Part model, mm, in its own coordinate system. Round coordinates to 2 decimals unless told otherwise and drop trailing zeros. Loops run counter-clockwise (first coordinate to the right, second up) from the corner with the lowest first, then second, coordinate; pieces in that order, holes last.
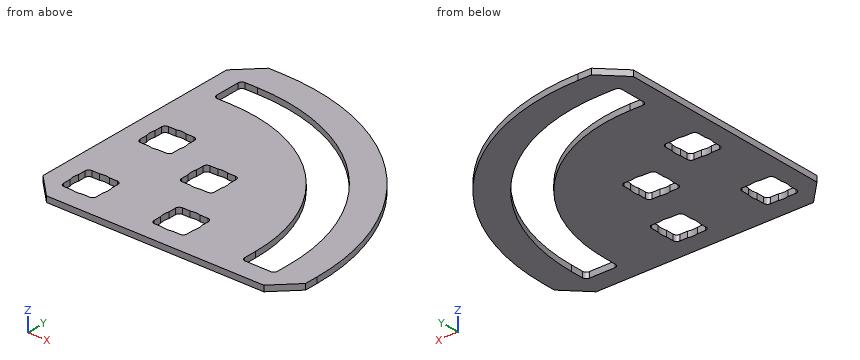
from build123d import *

# Parameters (mm, degrees)
BOSS_EXTRUDE1_DEPTH = 0.8128
SKETCH2_R           = 2.413
CUT_EXTRUDE1_DEPTH  = 2.54


with BuildPart() as part:
    # Sketch1 → Boss-Extrude1 (new body)
    with BuildSketch(Plane.XY.offset(0.8128)):
        with BuildLine():
            Line((-14.966560113, 23.146095061), (-14.966560113, -7.333904636))
            Line((-14.966560113, -7.333904636), (-11.791560113, -10.508904636))
            Line((-11.791560113, -10.508904636), (18.688439584, -10.508904636))
            Line((18.688439584, -10.508904636), (21.863439584, -7.333904636))
            Line((21.863439584, -7.333904636), (21.863439584, -5.428904939))
            ThreePointArc((21.863439584, -5.428904939), (12.564079886, 17.021735364), (-9.886560416, 26.321095061))
            Line((-9.886560416, 26.321095061), (-11.791560113, 26.321095061))
            Line((-11.791560113, 26.321095061), (-14.966560113, 23.146095061))
        make_face()
        with BuildLine():
            Line((17.316839733, -7.740304939), (13.710039804, -7.740304939))
            ThreePointArc((13.710039804, -7.740304939), (13.350829567, -7.591515187), (13.202039815, -7.23230495))
            Line((13.202039815, -7.23230495), (13.202039815, -5.428904939))
            ThreePointArc((13.202039815, -5.428904939), (6.439545376, 10.897200853), (-9.886560416, 17.659695293))
            Line((-9.886560416, 17.659695293), (-11.689960428, 17.659695293))
            ThreePointArc((-11.689960428, 17.659695293), (-12.049170664, 17.808485045), (-12.197960416, 18.167695282))
            Line((-12.197960416, 18.167695282), (-12.197960416, 21.77449521))
            ThreePointArc((-12.197960416, 21.77449521), (-12.049170664, 22.133705447), (-11.689960428, 22.282495199))
            Line((-11.689960428, 22.282495199), (-9.886560416, 22.282495199))
            ThreePointArc((-9.886560416, 22.282495199), (9.708358537, 14.166014015), (17.824839722, -5.428904939))
            Line((17.824839722, -5.428904939), (17.824839722, -7.23230495))
            ThreePointArc((17.824839722, -7.23230495), (17.67604997, -7.591515187), (17.316839733, -7.740304939))
        make_face(mode=Mode.SUBTRACT)
        with BuildLine():
            Line((5.124839584, -3.625504927), (5.124839584, -7.23230495))
            ThreePointArc((5.124839584, -7.23230495), (4.976049832, -7.591515187), (4.616839595, -7.740304939))
            Line((4.616839595, -7.740304939), (1.010039572, -7.740304939))
            ThreePointArc((1.010039572, -7.740304939), (0.650829336, -7.591515187), (0.502039584, -7.23230495))
            Line((0.502039584, -7.23230495), (0.502039584, -3.625504927))
            ThreePointArc((0.502039584, -3.625504927), (0.650829336, -3.266294691), (1.010039572, -3.117504939))
            Line((1.010039572, -3.117504939), (4.616839595, -3.117504939))
            ThreePointArc((4.616839595, -3.117504939), (4.976049832, -3.266294691), (5.124839584, -3.625504927))
        make_face(mode=Mode.SUBTRACT)
        with BuildLine():
            Line((-2.709790428, 5.862665061), (0.897009595, 5.862665061))
            ThreePointArc((0.897009595, 5.862665061), (1.256219832, 5.713875309), (1.405009584, 5.354665073))
            Line((1.405009584, 5.354665073), (1.405009584, 1.74786505))
            ThreePointArc((1.405009584, 1.74786505), (1.256219832, 1.388654813), (0.897009595, 1.239865061))
            Line((0.897009595, 1.239865061), (-2.709790428, 1.239865061))
            ThreePointArc((-2.709790428, 1.239865061), (-3.069000664, 1.388654813), (-3.217790416, 1.74786505))
            Line((-3.217790416, 1.74786505), (-3.217790416, 5.354665073))
            ThreePointArc((-3.217790416, 5.354665073), (-3.069000664, 5.713875309), (-2.709790428, 5.862665061))
        make_face(mode=Mode.SUBTRACT)
        with BuildLine():
            Line((-11.689960428, 9.582495061), (-8.083160405, 9.582495061))
            ThreePointArc((-8.083160405, 9.582495061), (-7.723950168, 9.433705309), (-7.575160416, 9.074495073))
            Line((-7.575160416, 9.074495073), (-7.575160416, 5.46769505))
            ThreePointArc((-7.575160416, 5.46769505), (-7.723950168, 5.108484813), (-8.083160405, 4.959695061))
            Line((-8.083160405, 4.959695061), (-11.689960428, 4.959695061))
            ThreePointArc((-11.689960428, 4.959695061), (-12.049170664, 5.108484813), (-12.197960416, 5.46769505))
            Line((-12.197960416, 5.46769505), (-12.197960416, 9.074495073))
            ThreePointArc((-12.197960416, 9.074495073), (-12.049170664, 9.433705309), (-11.689960428, 9.582495061))
        make_face(mode=Mode.SUBTRACT)
        with BuildLine():
            Line((-8.083160405, -7.740304939), (-11.689960428, -7.740304939))
            ThreePointArc((-11.689960428, -7.740304939), (-12.049170664, -7.591515187), (-12.197960416, -7.23230495))
            Line((-12.197960416, -7.23230495), (-12.197960416, -3.625504927))
            ThreePointArc((-12.197960416, -3.625504927), (-12.049170664, -3.266294691), (-11.689960428, -3.117504939))
            Line((-11.689960428, -3.117504939), (-8.083160405, -3.117504939))
            ThreePointArc((-8.083160405, -3.117504939), (-7.723950168, -3.266294691), (-7.575160416, -3.625504927))
            Line((-7.575160416, -3.625504927), (-7.575160416, -7.23230495))
            ThreePointArc((-7.575160416, -7.23230495), (-7.723950168, -7.591515187), (-8.083160405, -7.740304939))
        make_face(mode=Mode.SUBTRACT)
    extrude(amount=-BOSS_EXTRUDE1_DEPTH)

    # Sketch2 → Cut-Extrude1 (cut)
    with BuildSketch(Plane.XY.offset(0.8128)):
        with Locations((-9.886560416, 7.271095061)):
            Circle(SKETCH2_R)
        with Locations((-0.906390416, 3.551265061)):
            Circle(SKETCH2_R)
        with Locations((2.813439584, -5.428904939)):
            Circle(SKETCH2_R)
        with Locations((-9.886560416, -5.428904939)):
            Circle(SKETCH2_R)
    extrude(amount=-CUT_EXTRUDE1_DEPTH, mode=Mode.SUBTRACT)


solid = part.part
1) Slice it at C-C, the plane z = 0.2. Give the number of separate pieces and of enclosed holes in the cut face, then the cut area to 3 significant figures.
Values:
separate pieces: 1
enclosed holes: 5
area: 833 mm2
2) Wall check: line 1 along X through (y, z) = (6, 0.6); line 2 along X through (y, z) = (-7, 0.55); line 3 along Y through (x, z) = (2.5, 0.65). Give the ranges that are in metal, low to high.
Values:
line 1: x = -14.97 to -12.2, -7.58 to 10.17, 15.36 to 19.74
line 2: x = -14.97 to -12.2, -7.58 to 0.5, 5.12 to 13.2, 17.82 to 21.86
line 3: y = -10.51 to -7.82, -3.04 to 14.06, 19.36 to 23.81
3) Slice it at A-A, the plane x = 12. Give the cut face in (y, z).
Values:
outline: (-10.51, 0) - (1.92, 0) - (1.92, 0.81) - (-10.51, 0.81) - close; (11.57, 0) - (17.57, 0) - (17.57, 0.81) - (11.57, 0.81) - close
4) Slice it at B-B, the plane y = 15. Give the cut face in (x, z), then the cut area to 3 significant figures.
Values:
outline: (-14.97, 0) - (0.87, 0) - (0.87, 0.81) - (-14.97, 0.81) - close; (8.84, 0) - (14.42, 0) - (14.42, 0.81) - (8.84, 0.81) - close
area: 17.4 mm2
